```python
from build123d import *

# Parameters (mm, degrees)
BODY_EXTRUDE_DEPTH                       = 11.55
BODY_4_R                                 = 1.05
WINGS_CUT_EXTRUDE_DEPTH                  = 1.8
BODY_5_R                                 = 1.05
SCREW_HOLES_CUT_EXTRUDE_DEPTH            = 6
ADJUSTMENT_START                         = -15.995191
ADJUSTMENT_SCREW_HOLES_R                 = 2
ADJUSTMENT_SCREW_HOLES_CUT_EXTRUDE_DEPTH = 15.995191


with BuildPart() as part:
    # BODY → Body Extrude (new body)
    with BuildSketch(Plane.XY.offset(-35.57079385)):
        with BuildLine():
            Line((-3.75, -6.495190528), (-19.75, -6.495190528))
            Line((-19.75, -6.495190528), (-19.75, 9.5))
            Line((-19.75, 9.5), (19.75, 9.5))
            Line((19.75, 9.5), (19.75, -6.495190528))
            Line((19.75, -6.495190528), (3.75, -6.495190528))
            ThreePointArc((3.75, -6.495190528), (0, 7.5), (-3.75, -6.495190528))
        make_face()
    extrude(amount=-BODY_EXTRUDE_DEPTH)

    # BODY<4> → Wings Cut Extrude (cut)
    # profile 1 of 4: a face of its own
    with BuildSketch(Plane.XY.offset(-35.57079385)):
        with BuildLine():
            Line((10, 1.95), (7.242064623, 1.95))
            ThreePointArc((7.242064623, 1.95), (7.231272158, -1.98964896), (5.225169177, -5.380298047))
            Line((5.225169177, -5.380298047), (11.053, -1.641246782))
            ThreePointArc((11.053, -1.641246782), (11.711118056, -0.935187147), (11.95, 0))
            ThreePointArc((11.95, 0), (11.378858223, 1.378858223), (10, 1.95))
        make_face()
        with BuildLine():
            ThreePointArc((8.8, 0), (10, 1.2), (11.2, 0))
            ThreePointArc((11.2, 0), (10, -1.2), (8.8, 0))
        make_face(mode=Mode.SUBTRACT)
    # profile 2 of 4: a face of its own
    with BuildSketch(Plane.XY.offset(-35.57079385)):
        with BuildLine():
            ThreePointArc((11.2, 0), (10, -1.2), (8.8, 0))
            ThreePointArc((8.8, 0), (10, 1.2), (11.2, 0))
        make_face()
        with Locations((10, 0)):
            Circle(BODY_4_R, mode=Mode.SUBTRACT)
    # profile 3 of 4: a face of its own
    with BuildSketch(Plane.XY.offset(-35.57079385)):
        with BuildLine():
            Line((-11.053, -1.641246782), (-5.225169177, -5.380298047))
            ThreePointArc((-5.225169177, -5.380298047), (-7.231272158, -1.98964896), (-7.242064623, 1.95))
            Line((-7.242064623, 1.95), (-10, 1.95))
            ThreePointArc((-10, 1.95), (-11.871220354, 0.548666007), (-11.053, -1.641246782))
        make_face()
        with BuildLine():
            ThreePointArc((-11.2, 0), (-10, 1.2), (-8.8, 0))
            ThreePointArc((-8.8, 0), (-10, -1.2), (-11.2, 0))
        make_face(mode=Mode.SUBTRACT)
    # profile 4 of 4: a face of its own
    with BuildSketch(Plane.XY.offset(-35.57079385)):
        with BuildLine():
            ThreePointArc((-8.8, 0), (-10, -1.2), (-11.2, 0))
            ThreePointArc((-11.2, 0), (-10, 1.2), (-8.8, 0))
        make_face()
        with Locations((-10, 0)):
            Circle(BODY_4_R, mode=Mode.SUBTRACT)
    extrude(amount=-WINGS_CUT_EXTRUDE_DEPTH, mode=Mode.SUBTRACT)

    # BODY<5> → Screw Holes Cut Extrude (cut)
    with BuildSketch(Plane.XY.offset(-35.57079385)):
        with Locations((-10, 0)):
            Circle(BODY_5_R)
        with Locations((10, 0)):
            Circle(BODY_5_R)
    extrude(amount=-SCREW_HOLES_CUT_EXTRUDE_DEPTH, mode=Mode.SUBTRACT)

    # ADJUSTMENT SCREW HOLES → Adjustment Screw Holes Cut Extrude (cut)
    with BuildSketch(Plane(origin=(0, 9.5, 0), x_dir=(1, 0, 0), z_dir=(0, 1, 0)).offset(ADJUSTMENT_START)):
        with Locations(Location((-15.75, 41.49579385, 0), (0, 0, 270))):
            Circle(ADJUSTMENT_SCREW_HOLES_R)
        with Locations(Location((15.75, 41.49579385, 0), (0, 0, 270))):
            Circle(ADJUSTMENT_SCREW_HOLES_R)
    extrude(amount=ADJUSTMENT_SCREW_HOLES_CUT_EXTRUDE_DEPTH, mode=Mode.SUBTRACT)


solid = part.part
```
Build history of the part. All positions in model axes, mm. A direction names the side the tool comes from. Coordinates: 2 decimals unless noted, no trailing zeros. Order: outer loops, then holes, each group sorted by start corner. A loop starts at its lowest first (then second) coordinate and runs counter-clockwise, first axis right, second up.
Item 1: Drill centre lines: L1, parallel to X at y = 8.75, z = -42.5; L2, parallel to X at y = 0, z = -44; L3, parallel to X at y = 4, z = -40.75. Where is each one in solid material? Low to high.
Filled in:
L1: x = -19.75 to -17.48, -14.02 to 14.02, 17.48 to 19.75
L2: x = -19.75 to -7.5, 7.5 to 19.75
L3: x = -19.75 to -17.61, -13.89 to -6.34, 6.34 to 13.89, 17.61 to 19.75
Item 2: Saw through at A-A on y = 6. List the corners of the cut face in (x, z), then the cut area to 3 significant figures.
Filled in:
outline: (-19.75, -47.12) - (-4.5, -47.12) - (-4.5, -35.57) - (-19.75, -35.57) - close; (4.5, -47.12) - (19.75, -47.12) - (19.75, -35.57) - (4.5, -35.57) - close; hole circle Ø4 at (-15.75, -41.5); hole circle Ø4 at (15.75, -41.5)
area: 327 mm2
Item 3: Tool access for faces 1 (the flat face through (10, 0, -41.571)), 2 (the flat face through (19.75, 2, -41)): list every direction of +Z, -Z, +X, -X, +Y, -Y with a clear straight run to the whole face (end or side of a thin tool).
Filled in:
face 1: +Z
face 2: +Z, -Z, +X, +Y, -Y
Item 4: Saw through at B-B on z = -38. List the corners of the cut face in (x, y), then the cut area to 3 significant figures.
Filled in:
outline: (-19.75, -6.5) - (-3.75, -6.5) arc R7.5 cw (long way) to (3.75, -6.5) - (19.75, -6.5) - (19.75, 9.5) - (-19.75, 9.5) - close; hole circle Ø2.1 at (-10, 0); hole circle Ø2.1 at (10, 0)
area: 453 mm2
Item 5: Saw through at D-D on z = -40.75. List the corners of the cut face in (x, y), then the cut area to 3 significant figures.
Filled in:
outline: (-19.75, -6.5) - (-17.61, -6.5) - (-17.61, 9.5) - (-19.75, 9.5) - close; (-13.89, -6.5) - (-3.75, -6.5) arc R7.5 cw (long way) to (3.75, -6.5) - (13.89, -6.5) - (13.89, 9.5) - (-13.89, 9.5) - close; (17.61, -6.5) - (19.75, -6.5) - (19.75, 9.5) - (17.61, 9.5) - close; hole circle Ø2.1 at (-10, 0); hole circle Ø2.1 at (10, 0)
area: 335 mm2
Item 6: Saw through at C-C on x = 15.75. List the corners of the cut face in (y, z), then the cut area to 3 significant figures.
Filled in:
outline: (-6.5, -47.12) - (9.5, -47.12) - (9.5, -43.5) - (-6.5, -43.5) - close; (-6.5, -39.5) - (9.5, -39.5) - (9.5, -35.57) - (-6.5, -35.57) - close
area: 121 mm2
Item 7: Drop flat-ended pins along their axis: pin 1 Ø3.5 at (x, z) = (15.75, -41.5) entering from -Y; pin 2 Ø1.3 at (x, y) = (-10, 0) entering from +Z; pin 3 Ø2.5 at (x, y) = (10.5, 0) entering from +Z. Give the stop position or say it passes through.
Filled in:
pin 1: passes through
pin 2: stops at z = -41.57
pin 3: stops at z = -37.37
Item 8: Mould opens along Z. For faces 3 (the cylindrical face through (17.733, 1.39, -41.756)), 4 (the flat face through (-9, -1, -37.371)), 5 (the cylindrical face through (-14.4, 1.39, -42.97)), 6 (the flat face through (9, 1.95, -36)) say: released by +Z, released by -Z, zero draft, split by the parting line, or undercut.
Filled in:
face 3: undercut
face 4: released by +Z
face 5: undercut
face 6: zero draft
